```python
from build123d import *

# Parameters (mm, degrees)
SKETCH1_R           = 3
BOSS_EXTRUDE1_DEPTH = 10


with BuildPart() as part:
    # Sketch1 → Boss-Extrude1 (new body)
    with BuildSketch(Plane.XY):
        with BuildLine():
            Line((319.2, -227.34232335), (319.2, -20.84232335))
            ThreePointArc((319.2, -20.84232335), (334.2, -5.84232335), (319.2, 9.15767665))
            Line((319.2, 9.15767665), (319.2, 215.65767665))
            Line((319.2, 215.65767665), (228.3, 215.65767665))
            ThreePointArc((228.3, 215.65767665), (213.3, 230.65767665), (198.3, 215.65767665))
            Line((198.3, 215.65767665), (16.5, 215.65767665))
            ThreePointArc((16.5, 215.65767665), (1.5, 230.65767665), (-13.5, 215.65767665))
            Line((-13.5, 215.65767665), (-195.3, 215.65767665))
            ThreePointArc((-195.3, 215.65767665), (-210.3, 230.65767665), (-225.3, 215.65767665))
            Line((-225.3, 215.65767665), (-316.2, 215.65767665))
            Line((-316.2, 215.65767665), (-349.2, 187.967388821))
            Line((-349.2, 187.967388821), (-349.2, 9.15767665))
            ThreePointArc((-349.2, 9.15767665), (-364.2, -5.84232335), (-349.2, -20.84232335))
            Line((-349.2, -20.84232335), (-349.2, -199.652035521))
            Line((-349.2, -199.652035521), (-316.2, -227.34232335))
            Line((-316.2, -227.34232335), (-225.3, -227.34232335))
            ThreePointArc((-225.3, -227.34232335), (-210.3, -242.34232335), (-195.3, -227.34232335))
            Line((-195.3, -227.34232335), (-13.5, -227.34232335))
            ThreePointArc((-13.5, -227.34232335), (1.5, -242.34232335), (16.5, -227.34232335))
            Line((16.5, -227.34232335), (198.3, -227.34232335))
            ThreePointArc((198.3, -227.34232335), (213.3, -242.34232335), (228.3, -227.34232335))
            Line((228.3, -227.34232335), (319.2, -227.34232335))
        make_face()
        with Locations((-210.3, 223.15767665)):
            Circle(SKETCH1_R, mode=Mode.SUBTRACT)
        with Locations((1.5, 223.15767665)):
            Circle(SKETCH1_R, mode=Mode.SUBTRACT)
        with Locations((213.3, 223.15767665)):
            Circle(SKETCH1_R, mode=Mode.SUBTRACT)
        with Locations((326.7, -5.84232335)):
            Circle(SKETCH1_R, mode=Mode.SUBTRACT)
        with Locations((-356.7, -5.84232335)):
            Circle(SKETCH1_R, mode=Mode.SUBTRACT)
        with Locations((-210.3, -234.84232335)):
            Circle(SKETCH1_R, mode=Mode.SUBTRACT)
        with Locations((1.5, -234.84232335)):
            Circle(SKETCH1_R, mode=Mode.SUBTRACT)
        with Locations((213.3, -234.84232335)):
            Circle(SKETCH1_R, mode=Mode.SUBTRACT)
    extrude(amount=BOSS_EXTRUDE1_DEPTH)


solid = part.part
```
Source: CAD feature listing. Evaluate the final solid. Frame: model axes, mm. Give positions to 0.01 mm unless a question says otherwise; leave off trailing zeros. Order: outer loops, then holes, each group sorted by start corner. A loop starts at its lowest first (then second) coordinate and runs counter-clockwise, first axis right, second up.
(1) Section query C-C (y = 111). Return the cut outline in (x, z).
(2) Pull-direction query (X, two-part tool) for faces 1 (the face through (1.83, 230.654, 4.93)), 2 (the face through (334.196, -6.172, 4.93)), 3 (the face through (-364.196, -5.512, 4.93)); classes: +X half, -X half, draft (parallel to the pull), parting line (faces both ways), or undercut.
(3) Material intervals for line 1 along Y through (x, z) = (-210.3, 4.75); line 2 along X through (y, z) = (38, 2); line 3 along Y through (x, z) = (-26.5, 8.5), sorted ascending.
(4) Section query A-A (z = 4.25). State how many separate pieces and enclosed holes the cut face has, plus the area to 3 significant figures.
(5) Section query B-B (x = -244.5). Return the cut outline in (y, z).
(6) Contact query for flat-ended pins moving along their axis: P1, Ø9.5, axis at x = -210.3, y = -234.84, coming from the -Z side; P2, Ø5, axis at y = -87, z = 4.5, coming from the +X side; P3, Ø3, axis at y = 142.5, z = 6, coming from the -X side; P4, Ø3, axis at x = -113.5, z = 3, coming from the +Y side. Output: stop coordinate, or through.
Outcome:
1. outline: (-349.2, 0) - (319.2, 0) - (319.2, 10) - (-349.2, 10) - close
2. face 1: undercut
2. face 2: +X half
2. face 3: -X half
3. line 1: y = -242.34 to -237.84, -231.84 to 220.16, 226.16 to 230.66
3. line 2: x = -349.2 to 319.2
3. line 3: y = -227.34 to 215.66
4. separate pieces: 1
4. enclosed holes: 8
4. area: 298,000 mm2
5. outline: (-227.34, 0) - (215.66, 0) - (215.66, 10) - (-227.34, 10) - close
6. P1: stops at z = 0
6. P2: stops at x = 319.2
6. P3: stops at x = -349.2
6. P4: stops at y = 215.66
